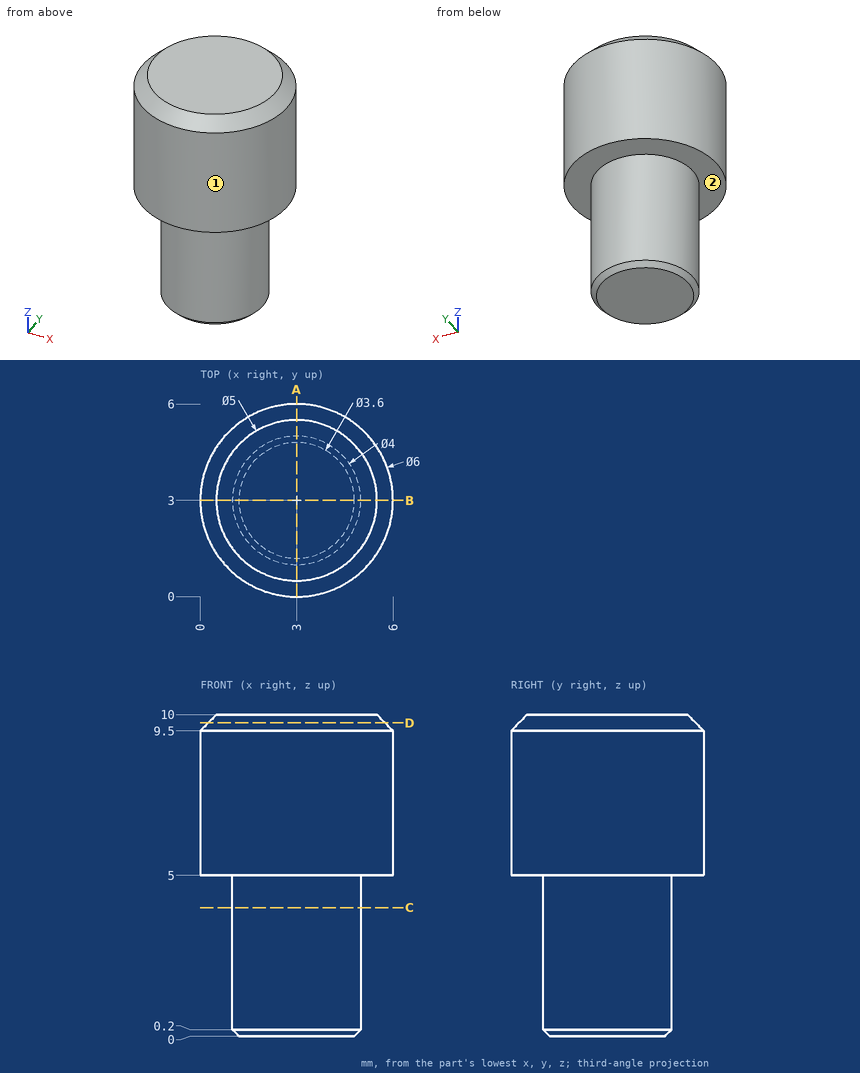
Study the drawing (mm; zero at the part's minimum x, y, z) and answer. A direction names the side the tool comes from. Give positions to 0.01 mm unless a question says otherwise; leave off trailing zeros. Write each loop counter-clockwise with the first axis right and the second up, starting at its lowest first coordinate (ties: lowest second). Pieces come first, ordered by that corner, then holes. Notation, with made-up numbers: (-2, 33.5) - (56, 33.5) arc R16 cw to (56, 51.5) - close; hole circle Ø1 at (-22.5, 9.25). An arc over 180 degrees is marked (long way). Write item = value, one per line. Start each with the question number.
Item 1: A tool of negligible diameter and unlimited length cuts with its end or side. For the marked faces 1 and 2, from which of +Z, -Z, +X, -X, +Y, -Y can it reach the whole face along a straight path? Write none if from no direction.
Item 2: Find section A-A (x = 3). Give the vertices of the cut face in (y, z), then the cut area to 3 significant figures.
Item 3: Find the intervals of material crossed by probe 1 along Z at (x, y) = (1, 4.3); probe 2 along X at (y, z) = (1.55, 9); probe 3 along Y at (x, z) = (3.25, 5.75), in increasing order. Write a range as [from, to].
Item 4: Find section D-D (z = 9.75). Give the vertices of the cut face in (x, y), then the cut area to 3 significant figures.
Item 5: Find section C-C (z = 4). Give the vertices of the cut face in (x, y).
Item 6: This flat-tipped pin is pushed along its axis until it touches: P1, Ø1, axis at x = 2, z = 7.5, coming from the -Y side. Where does it stop, or does it pass through?
Response:
q1.face_1 = +Z, -Z
q1.face_2 = -Z
q2.outline = (0, 5) - (1, 5) - (1, 0.2) - (1.2, 0) - (4.8, 0) - (5, 0.2) - (5, 5) - (6, 5) - (6, 9.5) - (5.5, 10) - (0.5, 10) - (0, 9.5) - close
q2.area = 49.7 mm²
q3.probe_1 = [5, 10]
q3.probe_2 = [0.37, 5.63]
q3.probe_3 = [0.01, 5.99]
q4.outline = circle Ø5.5 at (3, 3)
q4.area = 23.8 mm²
q5.outline = circle Ø4 at (3, 3)
q6.P1 = 0.04
